CAD build for the part. Positions are in the model's coordinates, mm. A direction names the side the tool comes from. Coordinates: 2 decimals unless noted, no trailing zeros. Loops run counter-clockwise (first coordinate to the right, second up) from the corner with the lowest first, then second, coordinate; pieces in that order, holes last. Notation, with made-up numbers: (68.25, -35) -> (121.25, -35) arc R15 ccw to (121.25, -24) -> close; hole circle Ø4 at (49.25, 80). An arc over 180 degrees is marked (long way). Answer as a JSON object with one key per item and string values. Group by question number.
from build123d import *

# Parameters (mm, degrees)
SKETCH1_W           = 63.5
SKETCH1_H           = 12.7
BOSS_EXTRUDE1_DEPTH = 76.2
SKETCH2_W           = 9.525
SKETCH2_H           = 3.175
BOSS_EXTRUDE2_DEPTH = 88.9
BOSS_EXTRUDE3_DEPTH = 3.175
BOSS_EXTRUDE4_DEPTH = 12.7


with BuildPart() as part:
    # Sketch1 → Boss-Extrude1 (new body)
    with BuildSketch(Plane(origin=(0, 0, 0), x_dir=(1, 0, 0), z_dir=(0, 1, 0))):
        Rectangle(SKETCH1_W, SKETCH1_H)
    extrude(amount=BOSS_EXTRUDE1_DEPTH)

    # Sketch2 → Boss-Extrude2 (add)
    with BuildSketch(Plane(origin=(0, 76.2, 0), x_dir=(1, 0, 0), z_dir=(0, 1, 0))):
        Rectangle(SKETCH2_W, SKETCH2_H)
        with Locations((-22.225, 0)):
            Rectangle(SKETCH2_W, SKETCH2_H)
        with Locations((22.225, 0)):
            Rectangle(SKETCH2_W, SKETCH2_H)
    extrude(amount=BOSS_EXTRUDE2_DEPTH)

    # Sketch3 → Boss-Extrude3 (add)
    with BuildSketch(Plane(origin=(0, 0, -1.5875), x_dir=(-1, 0, 0), z_dir=(0, 0, -1))):
        Polygon((-26.9875, 165.1), (-17.4625, 165.1), (-22.225, 169.300130206), align=None)
        Polygon((-4.7625, 165.1), (4.7625, 165.1), (0, 169.300130206), align=None)
        Polygon((17.4625, 165.1), (26.9875, 165.1), (22.225, 169.300130206), align=None)
    extrude(amount=-BOSS_EXTRUDE3_DEPTH)

    # Sketch4 → Boss-Extrude4 (add)
    with BuildSketch(Plane.XY.offset(6.35)):
        Polygon((31.75, 0), (0, -21.060567419), (-31.75, 0), align=None)
    extrude(amount=-BOSS_EXTRUDE4_DEPTH)


solid = part.part
Item 1: Band-saw the part on B-B, the plane z = 4.25. List the corners of the cut face in (x, y).
Item 2: Band-saw the part on C-C, the plane x = -13. List the corners of the cut face in (y, z).
Item 3: Band-saw the part on A-A, the plane y = 112. List the corners of the cut face in (x, z).
Item 4: Drill centre lines: L1, parallel to X at y = 137, z = -1; L2, parallel to Z at x = 26.5, y = 143.5; L3, parallel to Y at x = 7, z = 3.25. Where is each one in solid material? Low to high.
Item 5: 3-axis set-ups, long thin cutter, end or side, ignore diameter. For faces 1 (the flat face through (-2.415, 167.171, -0.022)), 2 (the flat face through (22, 123, -1.588)), 3 (the flat face through (26.988, 120, 0)), 4 (the flat face through (22, 123, 1.588)), 5 (the flat face through (-26.988, 120, 0)): which of +Z, -Z, +X, -X, +Y, -Y reach the whole face in a straight line?
Item 6: Pull direction X, two halves, no side cores. Call faces 6 (the flat face through (0, 122, -1.588)), 7 (the flat face through (-17.463, 120, 0)), 8 (the flat face through (-31.75, 38, 0)): +X half, -X half, draft (parallel to the pull), parting line (faces both ways), or undercut.
Item 7: Flat gauge pins, fed straight in: P1, Ø3.5, axis at y = 101, z = 0, coming from the -X side; P2, Ø3, axis at x = 22, y = 128, coming from the -Z side; P3, Ø3.5, axis at y = 118, z = -0.5, coming from the +X side. Where does each tip first touch, or does it go through?
Item 8: Band-saw the part on D-D, the plane y = -4. List the corners of the cut face in (x, z).
Reply:
{
 "1": {"outline": "(-31.75, 0) -> (0, -21.06) -> (31.75, 0) -> (31.75, 76.2) -> (-31.75, 76.2) -> close"},
 "2": {"outline": "(-12.44, -6.35) -> (76.2, -6.35) -> (76.2, 6.35) -> (-12.44, 6.35) -> close"},
 "3": {"outline": "(-26.99, -1.59) -> (-17.46, -1.59) -> (-17.46, 1.59) -> (-26.99, 1.59) -> close; (-4.76, -1.59) -> (4.76, -1.59) -> (4.76, 1.59) -> (-4.76, 1.59) -> close; (17.46, -1.59) -> (26.99, -1.59) -> (26.99, 1.59) -> (17.46, 1.59) -> close"},
 "4": {"L1": "-26.99 to -17.46, -4.76 to 4.76, 17.46 to 26.99", "L2": "-1.59 to 1.59", "L3": "-16.42 to 76.2"},
 "5": {"face 1": "+Z, -Z, +Y", "face 2": "-Z, +X, -X, +Y", "face 3": "+Z, -Z, +X, +Y", "face 4": "+Z, +X, -X, +Y", "face 5": "+Z, -Z, -X, +Y"},
 "6": {"face 6": "draft", "face 7": "undercut", "face 8": "-X half"},
 "7": {"P1": "x = -26.99", "P2": "z = -1.59", "P3": "x = 26.99"},
 "8": {"outline": "(-25.72, -6.35) -> (25.72, -6.35) -> (25.72, 6.35) -> (-25.72, 6.35) -> close"}
}
